Can you work these out from the drawing? Everything is in mm from the part's minimum corner. Round coordinates to 2 decimals unless told otherwise and drop trailing zeros. Loops run counter-clockwise (first coordinate to the right, second up) from the corner with the lowest first, then second, coordinate; pieces in that order, holes last. Notation, with made-up numbers: (-22.75, 51.5) -> (5.25, 51.5) arc R22 cw to (5.25, 84.5) -> close; hole circle Ø2 at (-3, 86). An arc over 180 degrees is marked (long way). One line per item, written item: value.
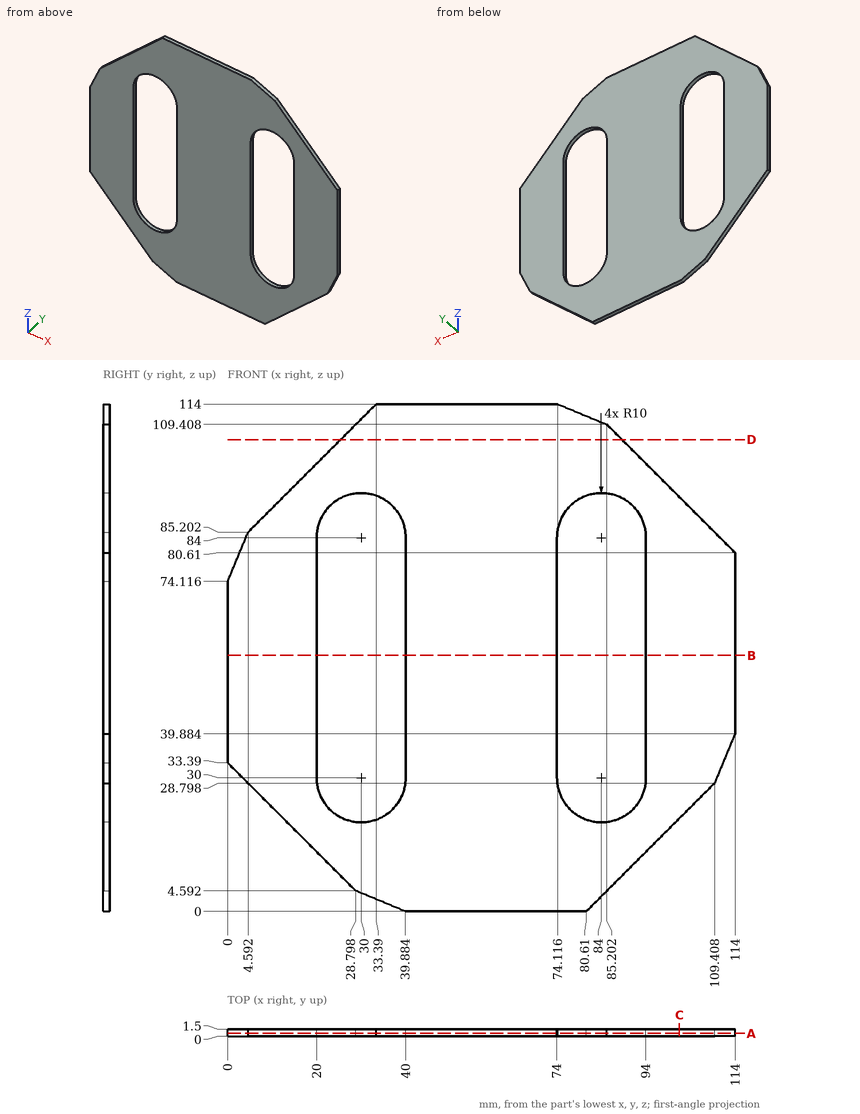
(1) Imagine slicing it at C-C on x = 101.5. Write out the boundary of the cut face in (y, z).
Results below:
outline: (0, 20.89) -> (1.5, 20.89) -> (1.5, 93.11) -> (0, 93.11) -> close
(2) For pin 1 Ø1.5 at (x, z) = (42, 102) entering from -Y, with a flat end and sliding along its axis, tell me the tip position at first contact or that it passes through.
Results below:
pin 1: stops at y = 0
(3) Imagine slicing it at B-B on z = 57.5. Write out the boundary of the cut face in (x, y).
Results below:
outline: (0, 0) -> (20, 0) -> (20, 1.5) -> (0, 1.5) -> close; (40, 0) -> (74, 0) -> (74, 1.5) -> (40, 1.5) -> close; (94, 0) -> (114, 0) -> (114, 1.5) -> (94, 1.5) -> close
(4) Imagine slicing it at D-D on z = 106. Write out the boundary of the cut face in (x, y).
Results below:
outline: (25.39, 0) -> (88.61, 0) -> (88.61, 1.5) -> (25.39, 1.5) -> close
(5) Imagine slicing it at A-A on y = 0.6. Write out the boundary of the cut face in (x, z) (1 decimal), then the cut area to 3 significant figures.
Results below:
outline: (0, 33.4) -> (28.8, 4.6) -> (39.9, 0) -> (80.6, 0) -> (109.4, 28.8) -> (114, 39.9) -> (114, 80.6) -> (85.2, 109.4) -> (74.1, 114) -> (33.4, 114) -> (4.6, 85.2) -> (0, 74.1) -> close; hole (20, 30) arc R10 ccw to (40, 30) -> (40, 84) arc R10 ccw to (20, 84) -> close; hole (74, 30) arc R10 ccw to (94, 30) -> (94, 84) arc R10 ccw to (74, 84) -> close
area: 7,920 mm²
(6) Please list where these lines run through material, in increasing order: L1, parallel to X at y = 0.4, z = 43.5; L2, parallel to X at y = 0.55, z = 90; L3, parallel to Z at x = 81, y = 0.95.
Results below:
L1: x = 0 to 20, 40 to 74, 94 to 114
L2: x = 9.39 to 22, 38 to 76, 92 to 104.61
L3: z = 0.39 to 20.46, 93.54 to 111.15
